Check sheet for the modelled part. Datum: model origin and axes. Units: mm. A direction names the side the tool comes from. Coordinates: 2 decimals unless noted, no trailing zeros. Loops run counter-clockwise (first coordinate to the right, second up) from the corner with the lowest first, then second, coordinate; pieces in that order, holes last. Notation, with made-up numbers: (10.25, 1.25) - (31.25, 1.25) arc R19 ccw to (31.25, 14.25) - close; hole circle Ø2 at (-29, -29.75). An arc over 180 degrees is marked (long way). Use a Markdown table: item, result. Add a question column.
1) Thickness scan on line 1 (Y direction, x = 0, z = 0.75); line 2 (X direction, y = 65, z = 2.2); line 3 (X direction, y = 64.5, z = 0.55). Record the ranges inside material, lowest first.
2) Sectioned sample at C-C, the plane y = 7.5. Enter the section's corners in (x, z), then the cut area to 3 significant figures.
3) Sectioned sample at D-D, the plane x = -12.5. Enter the section's corners in (y, z), then the cut area to 3 significant figures.
4) Sectioned sample at A-A, the plane x = 0. Enter the section's corners in (y, z).
5) Draft check along X on faces 3 (the flat face through (-10, 45, 1)), 4 (the flat face through (0, 27, 3)), 5 (the flat face through (-21.64, 17.89, 1.48)). Enter one of: pulls with the +X half, pulls with the -X half, needs draft (parallel to the pull), parting line crosses it, or undercut.
6) Go/stop test with a flat-tipped pin: P1, Ø0.9, axis at y = 44.5, z = 1.5, coming from the -X side. Record where the tip stops, or that it passes through.
7) Tool access check on faces 1 (the cylindrical face through (0, -20, 1)), 2 (the flat face through (10, 45, 1)). Record the directions out of +Z, -Z, +X, -X, +Y, -Y that give a thin tool (end or side, any length) a straight path to the whole face; none if there is none.
8) Sectioned sample at B-B, the plane z = 0.6. Enter the section's corners in (x, y), then the cut area to 3 significant figures.
from build123d import *

# Parameters (mm, degrees)
SKETCH_1_R      = 1.5
SKETCH_1_R_2    = 13.5
EXTRUDE_1_DEPTH = 3
FILLET_2_R      = 1


with BuildPart() as part:
    # 草图1 → 凸台-拉伸1 (new body)
    with BuildSketch(Plane.XY):
        with BuildLine():
            Line((-32.4, 72.5), (32.4, 72.5))
            Line((32.4, 72.5), (32.4, 57.5))
            Line((32.4, 57.5), (23.422667354, 38.248048013))
            Line((23.422667354, 38.248048013), (19.923893962, -1.743114855))
            ThreePointArc((19.923893962, -1.743114855), (0, -20), (-19.923893962, -1.743114855))
            Line((-19.923893962, -1.743114855), (-23.422667354, 38.248048013))
            Line((-23.422667354, 38.248048013), (-32.4, 57.5))
            Line((-32.4, 57.5), (-32.4, 72.5))
        make_face()
        with Locations((25, 65)):
            Circle(SKETCH_1_R, mode=Mode.SUBTRACT)
        with Locations((-25, 65)):
            Circle(SKETCH_1_R, mode=Mode.SUBTRACT)
        with Locations((0, 65)):
            Circle(SKETCH_1_R, mode=Mode.SUBTRACT)
        Circle(SKETCH_1_R_2, mode=Mode.SUBTRACT)
        with Locations((-9, 25)):
            Circle(SKETCH_1_R, mode=Mode.SUBTRACT)
        with Locations((9, 25)):
            Circle(SKETCH_1_R, mode=Mode.SUBTRACT)
        with BuildLine():
            Line((10, 47.5), (10, 42.5))
            ThreePointArc((10, 42.5), (0, 32.5), (-10, 42.5))
            Line((-10, 42.5), (-10, 47.5))
            ThreePointArc((-10, 47.5), (0, 57.5), (10, 47.5))
        make_face(mode=Mode.SUBTRACT)
    extrude(amount=EXTRUDE_1_DEPTH)

    # 圆角2
    fillet_2_edges = [part.edges().sort_by_distance(p)[0] for p in [
        (23.422667354, 38.248048013, 1.5),
        (-23.422667354, 38.248048013, 1.5),
        (-32.4, 57.5, 1.5),
        (-32.4, 72.5, 1.5),
        (32.4, 72.5, 1.5),
        (32.4, 57.5, 1.5),
    ]]
    fillet(fillet_2_edges, radius=FILLET_2_R)


solid = part.part
Solved:
| question | item | result |
|---|---|---|
| 1 | line 1 | y = -20 to -13.5, 13.5 to 32.5, 57.5 to 63.5, 66.5 to 72.5 |
| 1 | line 2 | x = -32.4 to -26.5, -23.5 to -1.5, 1.5 to 23.5, 26.5 to 32.4 |
| 1 | line 3 | x = -32.4 to -26.41, -23.59 to -1.41, 1.41 to 23.59, 26.41 to 32.4 |
| 2 | outline | (-20.73, 0) - (-11.22, 0) - (-11.22, 3) - (-20.73, 3) - close; (11.22, 0) - (20.73, 0) - (20.73, 3) - (11.22, 3) - close |
| 2 | area | 57.0 mm2 |
| 3 | outline | (-15.61, 0) - (-5.1, 0) - (-5.1, 3) - (-15.61, 3) - close; (5.1, 0) - (72.5, 0) - (72.5, 3) - (5.1, 3) - close |
| 3 | area | 234 mm2 |
| 4 | outline | (-20, 0) - (-13.5, 0) - (-13.5, 3) - (-20, 3) - close; (13.5, 0) - (32.5, 0) - (32.5, 3) - (13.5, 3) - close; (57.5, 0) - (63.5, 0) - (63.5, 3) - (57.5, 3) - close; (66.5, 0) - (72.5, 0) - (72.5, 3) - (66.5, 3) - close |
| 5 | face 3 | undercut |
| 5 | face 4 | needs draft |
| 5 | face 5 | pulls with the -X half |
| 6 | P1 | stops at x = -26.55 |
| 7 | face 1 | +Z, -Z, -Y |
| 7 | face 2 | +Z, -Z |
| 8 | outline | (-32.4, 57.72) arc R1 ccw to (-32.31, 57.3) - (-23.5, 38.41) arc R1 cw to (-23.41, 38.07) - (-19.92, -1.74) arc R20 ccw to (19.92, -1.74) - (23.41, 38.07) arc R1 cw to (23.5, 38.41) - (32.31, 57.3) arc R1 ccw to (32.4, 57.72) - (32.4, 71.5) arc R1 ccw to (31.4, 72.5) - (-31.4, 72.5) arc R1 ccw to (-32.4, 71.5) - close; hole circle Ø3 at (-25, 65); hole circle Ø27 at (0, 0); hole circle Ø3 at (-9, 25); hole (-10, 42.5) arc R10 ccw to (10, 42.5) - (10, 47.5) arc R10 ccw to (-10, 47.5) - close; hole circle Ø3 at (0, 65); hole circle Ø3 at (9, 25); hole circle Ø3 at (25, 65) |
| 8 | area | 3,320 mm2 |
